from build123d import *

# Parameters (mm, degrees)
CROQUIS1_W              = 10
CROQUIS1_H              = 10
SALIENTE_EXTRUIR1_DEPTH = 1
SALIENTE_EXTRUIR2_DEPTH = 1


with BuildPart() as part:
    # Croquis1 → Saliente-Extruir1 (new body)
    with BuildSketch(Plane.XY):
        Rectangle(CROQUIS1_W, CROQUIS1_H)
    extrude(amount=SALIENTE_EXTRUIR1_DEPTH)

    # Croquis2 → Saliente-Extruir2 (add, through all)
    with BuildSketch(Plane.XY.offset(1)):
        with BuildLine():
            Line((-5, 5), (-5.125, 5))
            ThreePointArc((-5.125, 5), (-6.539213562, 4.414213562), (-7.125, 3))
            Line((-7.125, 3), (-7.125, 2.75))
            Line((-7.125, 2.75), (-5, 2.75))
            Line((-5, 2.75), (-5, 5))
        make_face()
        with BuildLine():
            Line((5, 2.75), (7.125, 2.75))
            Line((7.125, 2.75), (7.125, 3))
            ThreePointArc((7.125, 3), (6.539213562, 4.414213562), (5.125, 5))
            Line((5.125, 5), (5, 5))
            Line((5, 5), (5, 2.75))
        make_face()
        with BuildLine():
            Line((5, -5), (5.125, -5))
            ThreePointArc((5.125, -5), (6.539213562, -4.414213562), (7.125, -3))
            Line((7.125, -3), (7.125, -2.75))
            Line((7.125, -2.75), (5, -2.75))
            Line((5, -2.75), (5, -5))
        make_face()
        with BuildLine():
            Line((-5, -2.75), (-7.125, -2.75))
            Line((-7.125, -2.75), (-7.125, -3))
            ThreePointArc((-7.125, -3), (-6.539213562, -4.414213562), (-5.125, -5))
            Line((-5.125, -5), (-5, -5))
            Line((-5, -5), (-5, -2.75))
        make_face()
    extrude(amount=-SALIENTE_EXTRUIR2_DEPTH)


solid = part.part
Input: part model. Units: mm. Frame: model coordinates. A direction names the side the tool comes from. Give positions to 0.01 mm unless a question says otherwise; leave off trailing zeros. Loops run counter-clockwise (first coordinate to the right, second up) from the corner with the lowest first, then second, coordinate; pieces in that order, holes last. Notation, with made-up numbers: (74, -9.5) -> (128, -9.5) arc R18 cw to (128, 12.5) -> close; hole circle Ø3 at (58.25, 31.5). An arc over 180 degrees is marked (long way). Answer as a JSON object with one key per item and string values. Group by question number.
Item 1: Pin query (flat end, axial travel): P1, Ø0.5, axis at y = 0, z = 0.5, coming from the +X side. Return the tip coordinate at first contact, or that it passes through.
Item 2: Cut plane A-A, the plane x = 5.5. Return the cut outline in (y, z), and give its area (3 significant figures).
Item 3: Cut plane C-C, the plane y = 2. Return the cut outline in (x, z).
Item 4: Cut plane D-D, the plane y = 4.25. Return the cut outline in (x, z).
Item 5: Cut plane B-B, the plane z = 0.5. Return the cut outline in (x, y) (3 decimals).
Item 6: Line query: probe 1 along X at (y, z) = (2.5, 0.9); probe 2 along X at (y, z) = (-3.25, 0.1); probe 3 along Y at (x, z) = (-5.5, 0.6). Output: solid intervals per line, ascending.
Item 7: Reachability of faces 1 (the flat face through (6, 2.75, 0.5)), 2 (the flat face through (0.1, 5, 0.5)), 3 (the flat face through (-5, 0, 0.5)) from +Z, -Z, +X, -X, +Y, -Y: full face, straight path, thin tool, end or side. Return the list, or none.
Checks:
{
 "1": {"P1": "stops at x = 5"},
 "2": {"outline": "(-4.96, 0) -> (-2.75, 0) -> (-2.75, 1) -> (-4.96, 1) -> close; (2.75, 0) -> (4.96, 0) -> (4.96, 1) -> (2.75, 1) -> close", "area": "4.43 mm²"},
 "3": {"outline": "(-5, 0) -> (5, 0) -> (5, 1) -> (-5, 1) -> close"},
 "4": {"outline": "(-6.69, 0) -> (6.69, 0) -> (6.69, 1) -> (-6.69, 1) -> close"},
 "5": {"outline": "(-7.125, -3) arc R2 ccw to (-5.125, -5) -> (5.125, -5) arc R2 ccw to (7.125, -3) -> (7.125, -2.75) -> (5, -2.75) -> (5, 2.75) -> (7.125, 2.75) -> (7.125, 3) arc R2 ccw to (5.125, 5) -> (-5.125, 5) arc R2 ccw to (-7.125, 3) -> (-7.125, 2.75) -> (-5, 2.75) -> (-5, -2.75) -> (-7.125, -2.75) -> close"},
 "6": {"probe 1": "x = -5 to 5", "probe 2": "x = -7.11 to 7.11", "probe 3": "y = -4.96 to -2.75, 2.75 to 4.96"},
 "7": {"face 1": "+Z, -Z, +X", "face 2": "+Z, -Z, +X, -X, +Y", "face 3": "+Z, -Z, -X"}
}
